```python
from build123d import *

# Parameters (mm, degrees)
SKETCH1_R           = 9.25
BOSS_EXTRUDE1_DEPTH = 55
SKETCH2_W           = 11
SKETCH2_H           = 3.5
CUT_EXTRUDE1_DEPTH  = 51
CHAMFER1_SIZE       = 0.8
SKETCH3_R           = 2.5
CUT_EXTRUDE2_DEPTH  = 10
SKETCH5_W           = 6
SKETCH5_H           = 2.5
BOSS_EXTRUDE2_DEPTH = 20
SKETCH6_W           = 6
SKETCH6_H           = 2.5
BOSS_EXTRUDE3_DEPTH = 10
SKETCH8_W           = 8
SKETCH8_H           = 3
CUT_EXTRUDE3_DEPTH  = 10


with BuildPart() as part:
    # Sketch1 → Boss-Extrude1 (new body)
    with BuildSketch(Plane(origin=(0, 0, 0), x_dir=(1, 0, 0), z_dir=(0, 1, 0))):
        with Locations(Location((0, 0, 0), (0, 0, 270))):
            Circle(SKETCH1_R)
    extrude(amount=BOSS_EXTRUDE1_DEPTH)

    # Sketch2 → Cut-Extrude1 (cut)
    with BuildSketch(Plane(origin=(0, 55, 0), x_dir=(1, 0, 0), z_dir=(0, 1, 0))):
        Rectangle(SKETCH2_W, SKETCH2_H)
    extrude(amount=-CUT_EXTRUDE1_DEPTH, mode=Mode.SUBTRACT)

    # Chamfer1
    chamfer1_edges = [part.edges().sort_by_distance(p)[0] for p in [
        (5.5, 55, 0),
        (0, 55, -1.75),
        (-5.5, 55, 0),
        (0, 55, 1.75),
    ]]
    chamfer(chamfer1_edges, length=CHAMFER1_SIZE)

    # Sketch3 → Cut-Extrude2 (cut)
    with BuildSketch(Plane.XY.offset(10)):
        with Locations((0, 43)):
            Circle(SKETCH3_R)
        with Locations((0, 35)):
            Circle(SKETCH3_R)
        with Locations((0, 27)):
            Circle(SKETCH3_R)
        with Locations((0, 19)):
            Circle(SKETCH3_R)
        with Locations((0, 11)):
            Circle(SKETCH3_R)
    extrude(amount=-CUT_EXTRUDE2_DEPTH, mode=Mode.SUBTRACT)

    # Sketch5 → Boss-Extrude2 (add)
    with BuildSketch(Plane(origin=(18, 0, 0), x_dir=(0, 0, -1), z_dir=(1, 0, 0))):
        with Locations((0, 1.25)):
            Rectangle(SKETCH5_W, SKETCH5_H)
    extrude(amount=-BOSS_EXTRUDE2_DEPTH)

    # Sketch6 → Boss-Extrude3 (add)
    with BuildSketch(Plane(origin=(-18, 0, 0), x_dir=(0, 0, -1), z_dir=(1, 0, 0))):
        with Locations((0, 1.25)):
            Rectangle(SKETCH6_W, SKETCH6_H)
    extrude(amount=BOSS_EXTRUDE3_DEPTH)

    # Sketch8 → Cut-Extrude3 (cut)
    with BuildSketch(Plane.XZ):
        with Locations((14, 1.5)):
            Rectangle(SKETCH8_W, SKETCH8_H)
        with Locations((-14, -1.5)):
            Rectangle(SKETCH8_W, SKETCH8_H)
    extrude(amount=-CUT_EXTRUDE3_DEPTH, mode=Mode.SUBTRACT)


solid = part.part
```
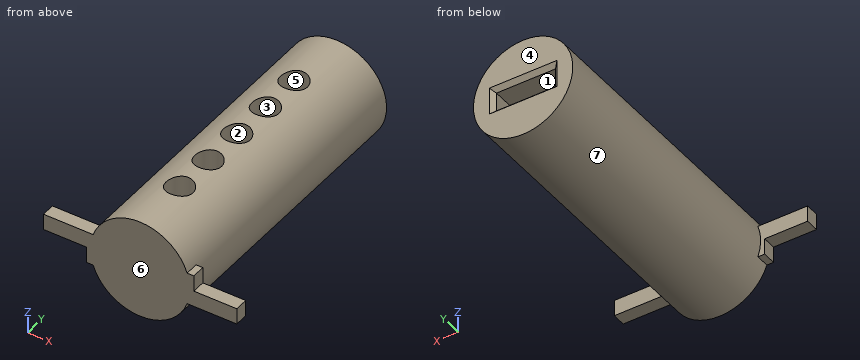
Work out the finished part from the listing and answer in its coordinate system (mm). Face numbers are marked on the shaded views. A direction names the side the tool comes from. Give positions to 0.01 mm unless a question says otherwise; leave off trailing zeros. Loops run counter-clockwise (first coordinate to the right, second up) from the corner with the lowest first, then second, coordinate; pieces in that order, holes last. Notation, with made-up numbers: M 6.25,-26 L 65.25,-26 A29 ccw 65.25,3 Z; hole C 89,-24 d7. An arc over 180 degrees is marked long. One line per item, written item: value. Start each with the question number.
1. Which of the six approach directions +Z, -Z, +X, -X, +Y, -Y give full straight-line access (tool end or side, diameter ignored) to the marked faces 5, 6 and 7?
2. Find section A-A (x = 0). State how many separate pieces and enclosed holes the cut face has, and give its area (3 significant figures).
3. Find the intervals of material crossed by probe 1 along Y at (x, z) = (0, 6.75); probe 2 along X at (y, z) = (10.5, 8.25); probe 3 along X at (y, z) = (43.5, 1), in increasing order.
4. Determine the mould class of the marked faces 1, 2, 3 and 4 for opening direction Y: released by +Y, released by -Y, zero draft, split by the parting line, or undercut.
5. Find section D-D (y = 35). Give the vertices of the cut face in (x, z), and give its area (3 significant figures).
6. Find section B-B (z = 7.25). Give the vertices of the cut face in (x, y), and give its area (3 significant figures).
7. Find section C-C (y = 49.5). Give the vertices of the cut face in (x, z).
8. Each of these flat-tipped pins is pushed along its axis until it touches: P1, Ø4, axis at y = 43.5, z = -3.5, coming from the -X side; P2, Ø3, axis at y = 16, z = 3, coming from the +X side; P3, Ø3, axis at y = 1.5, z = -2, coming from the -X side. Where does it stop, or does it pass through?
Reported:
1. face 5: +Z
1. face 6: +Z, -Z, +X, -X, -Y
1. face 7: +Y
2. separate pieces: 6
2. enclosed holes: 0
2. area: 651 mm²
3. probe 1: y = 0 to 8.5, 13.5 to 16.5, 21.5 to 24.5, 29.5 to 32.5, 37.5 to 40.5, 45.5 to 55
3. probe 2: x = -4.18 to -2.45, 2.45 to 4.18
3. probe 3: x = -9.2 to -5.5, 5.5 to 9.2
4. face 1: zero draft
4. face 2: undercut
4. face 3: undercut
4. face 4: released by +Y
5. outline: M -5.5,-1.75 L -5.5,1.75 L -2.5,1.75 L -2.5,8.91 A9.25 ccw long 2.5,8.91 L 2.5,1.75 L 5.5,1.75 L 5.5,-1.75 Z
5. area: 193 mm²
6. outline: M -5.74,0 L 5.74,0 L 5.74,55 L -5.74,55 Z; hole C 0,11 d5; hole C 0,19 d5; hole C 0,27 d5; hole C 0,35 d5; hole C 0,43 d5
6. area: 534 mm²
7. outline: C 0,0 d18.5; hole M -5.5,-1.75 L 5.5,-1.75 L 5.5,1.75 L -5.5,1.75 Z
8. P1: stops at x = -9.13
8. P2: stops at x = 9.13
8. P3: stops at x = -10
